Print and shaded views of the part. All mm, measured from the part's lowest x, y and z. A direction names the side the tool comes from. Coordinates: 2 decimals unless noted, no trailing zeros. Loops run counter-clockwise (first coordinate to the right, second up) from the corner with the lowest first, then second, coordinate; pieces in that order, holes last.
1) Which spindle directions (+Z, -Z, +X, -X, +Y, -Y) get a long thin tool onto all of the face, cutting with end or side? Do the marked faces 5, 6 and 7. Say none if no direction does.
2) Pin check, flat tips, straight feed: pin 1 Ø1.5 at (x, z) = (1, 5) entering from -Y; pin 2 Ø12 at (y, z) = (12.5, 20) entering from +X; pin 3 Ø1.6 at (x, y) = (22, 3) entering from +Z; pin 4 Ø1.6 at (y, z) = (64, 12) entering from -X. Stop position of each tip, or through.
3) Saw through at D-D, the plane z = 14. Write the cut outline in (x, y).
4) Saw through at C-C, the plane x = 12.75. Write the cut outline in (y, z), and give its area (3 significant figures).
5) Saw through at A-A, the plane z = 25. Write the cut outline in (x, y), and give its area (3 significant figures).
6) Two-plate mould, pull along Y, no slides. Class the marked faces 1, 2, 3 and 4: +Y half, -Y half, draft (parallel to the pull), parting line (faces both ways), or undercut.
7) Wall check: line 1 along Y through (x, z) = (2, 22.5); line 2 along X through (y, z) = (3, 9.5); line 3 along Y through (x, z) = (8, 13). Give the ranges that are in metal, low to high.
8) Saw through at B-B, the plane y = 54. Write the cut outline in (x, z), and give its area (3 significant figures).
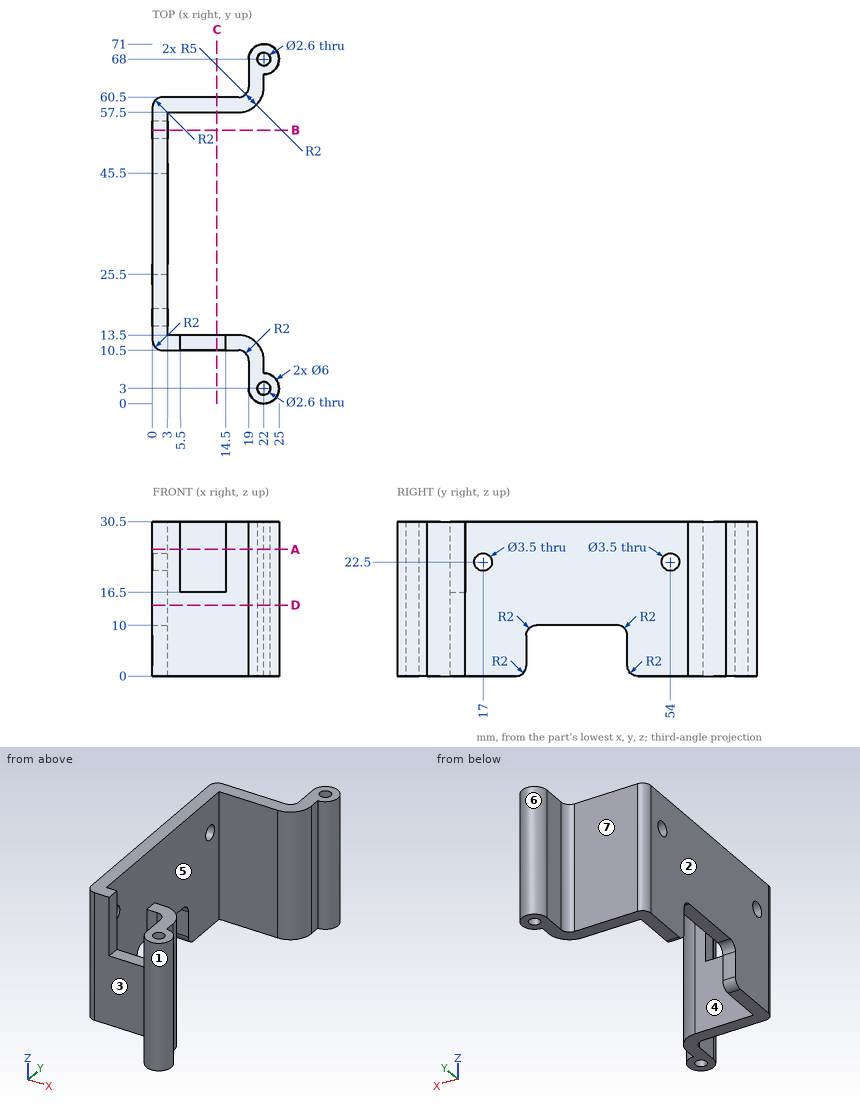
Data:
1. face 5: +Z, -Z, +X
1. face 6: +Z, -Z
1. face 7: +Z, -Z, -X, +Y
2. pin 1: stops at y = 10.52
2. pin 2: stops at x = 22
2. pin 3: passes through
2. pin 4: stops at x = 19
3. outline: (0, 12.5) arc R2 ccw to (2, 10.5) - (17, 10.5) arc R2 cw to (19, 8.5) - (19, 3) arc R3 ccw (long way) to (22, 6) - (22, 8.5) arc R5 ccw to (17, 13.5) - (3, 13.5) - (3, 57.5) - (17, 57.5) arc R5 ccw to (22, 62.5) - (22, 65) arc R3 ccw (long way) to (19, 68) - (19, 62.5) arc R2 cw to (17, 60.5) - (2, 60.5) arc R2 ccw to (0, 58.5) - close; hole circle Ø2.6 at (22, 3); hole circle Ø2.6 at (22, 68)
4. outline: (10.5, 0) - (13.5, 0) - (13.5, 16.5) - (10.5, 16.5) - close; (57.5, 0) - (60.5, 0) - (60.5, 30.5) - (57.5, 30.5) - close
4. area: 141 mm2
5. outline: (0, 12.5) arc R2 ccw to (2, 10.5) - (5.5, 10.5) - (5.5, 13.5) - (3, 13.5) - (3, 57.5) - (17, 57.5) arc R5 ccw to (22, 62.5) - (22, 65) arc R3 ccw (long way) to (19, 68) - (19, 62.5) arc R2 cw to (17, 60.5) - (2, 60.5) arc R2 ccw to (0, 58.5) - close; (14.5, 10.5) - (17, 10.5) arc R2 cw to (19, 8.5) - (19, 3) arc R3 ccw (long way) to (22, 6) - (22, 8.5) arc R5 ccw to (17, 13.5) - (14.5, 13.5) - close; hole circle Ø2.6 at (22, 3); hole circle Ø2.6 at (22, 68)
5. area: 303 mm2
6. face 1: undercut
6. face 2: draft
6. face 3: -Y half
6. face 4: undercut
7. line 1: y = 10.5 to 15.25, 18.75 to 52.25, 55.75 to 60.5
7. line 2: x = 19 to 20.7, 23.3 to 25
7. line 3: y = 10.5 to 13.5, 57.5 to 60.5
8. outline: (0, 0) - (3, 0) - (3, 20.75) - (0, 20.75) - close; (0, 24.25) - (3, 24.25) - (3, 30.5) - (0, 30.5) - close
8. area: 81.0 mm2
